```python
from build123d import *

# Parameters (mm, degrees)
SKETCH1_R           = 1.55
BOSS_EXTRUDE1_DEPTH = 4
SKETCH2_W           = 60
SKETCH2_H           = 8
BOSS_EXTRUDE2_DEPTH = 5


with BuildPart() as part:
    # Sketch1 → Boss-Extrude1 (new body)
    with BuildSketch(Plane.XY):
        Polygon((-30, 56), (-30, -56), (-10, -56), (-10, -36), (10, -36), (10, -56), (30, -56), (30, 56), align=None)
        with Locations((-20, -46)):
            Circle(SKETCH1_R, mode=Mode.SUBTRACT)
        with Locations((20, -46)):
            Circle(SKETCH1_R, mode=Mode.SUBTRACT)
        with Locations((-20, 46)):
            Circle(SKETCH1_R, mode=Mode.SUBTRACT)
        with Locations((20, 46)):
            Circle(SKETCH1_R, mode=Mode.SUBTRACT)
    extrude(amount=BOSS_EXTRUDE1_DEPTH)

    # Sketch2 → Boss-Extrude2 (add)
    with BuildSketch(Plane(origin=(0, 0, 0), x_dir=(-1, 0, 0), z_dir=(0, 0, -1))):
        with Locations((0, 32)):
            Rectangle(SKETCH2_W, SKETCH2_H)
        Polygon((30, -28), (-30, -28), (-30, -36), (-10, -36), (10, -36), (30, -36), align=None)
    extrude(amount=BOSS_EXTRUDE2_DEPTH)


solid = part.part
```
For this review, take the finished solid that the model builds, in its own axes (mm). A direction names the side the tool comes from. Round coordinates to 2 decimals unless told otherwise and drop trailing zeros. Order: outer loops, then holes, each group sorted by start corner. A loop starts at its lowest first (then second) coordinate and runs counter-clockwise, first axis right, second up. Notation, with made-up numbers: (86.5, 48) -> (110.5, 48) arc R22 ccw to (110.5, 65) -> close; hole circle Ø4 at (-35, 42.25). An arc over 180 degrees is marked (long way). Use a Markdown table: item, result.
Item 1: Machinability: for faces 4 (the flat face through (0, 36, -2)), 5 (the flat face through (0, -28, -2)), 6 (the flat face through (18, -46, 0)), 7 (the flat face through (-10, -46, 2)), which of the approach directions +Z, -Z, +X, -X, +Y, -Y give a long, thin tool a straight path to every point of the face, cutting with its end or side? Answer none if there is none.
Resolved:
| item | result |
|---|---|
| face 4 | -Z, +X, -X, +Y |
| face 5 | -Z, +X, -X |
| face 6 | -Z, +X, -X, -Y |
| face 7 | +Z, -Z, -Y |
Item 2: Take a section at B-B (x = -20). State the section outline as (y, z) points, plus the area to 3 significant figures.
Resolved:
| item | result |
|---|---|
| outline | (-56, 0) -> (-47.55, 0) -> (-47.55, 4) -> (-56, 4) -> close; (-44.45, 0) -> (-36, 0) -> (-36, -5) -> (-28, -5) -> (-28, 0) -> (28, 0) -> (28, -5) -> (36, -5) -> (36, 0) -> (44.45, 0) -> (44.45, 4) -> (-44.45, 4) -> close; (47.55, 0) -> (56, 0) -> (56, 4) -> (47.55, 4) -> close |
| area | 503 mm² |
Item 3: Take a section at A-A (z = -3). State the section outline as (x, y) points, plus the area to 3 significant figures.
Resolved:
| item | result |
|---|---|
| outline | (-30, -36) -> (30, -36) -> (30, -28) -> (-30, -28) -> close; (-30, 28) -> (30, 28) -> (30, 36) -> (-30, 36) -> close |
| area | 960 mm² |
Item 4: For pin 1 (5 mm diameter, centred on x = -20, y = -46, fed in from +Z); pin 2 (10 mm diameter, centred on x = 8.5, y = -4, fed in from -Z); pin 3 (2.5 mm diameter, centred on x = 4.5, z = -2, fed in from +Y); pin 4 (1.5 mm diameter, centred on x = 12, z = -3.5, fed in from -Y), all flat-tipped, find the tip position at first contact; note any pin that passes through.
Resolved:
| item | result |
|---|---|
| pin 1 | stops at z = 4 |
| pin 2 | stops at z = 0 |
| pin 3 | stops at y = 36 |
| pin 4 | stops at y = -36 |
Item 5: For line 1 along Y through (x, z) = (-20, 1.55); line 2 along Y through (x, z) = (-4.5, -1); line 3 along Z through (x, y) = (4.5, -22), list the stretches that pass through material, from the lowest coordinate up. Write a range as [from, to].
Resolved:
| item | result |
|---|---|
| line 1 | y = [-56, -47.55], [-44.45, 44.45], [47.55, 56] |
| line 2 | y = [-36, -28], [28, 36] |
| line 3 | z = [0, 4] |
Item 6: Take a section at D-D (z = 2.25). State the section outline as (x, y) points, plus the area to 3 significant figures.
Resolved:
| item | result |
|---|---|
| outline | (-30, -56) -> (-10, -56) -> (-10, -36) -> (10, -36) -> (10, -56) -> (30, -56) -> (30, 56) -> (-30, 56) -> close; hole circle Ø3.1 at (-20, -46); hole circle Ø3.1 at (-20, 46); hole circle Ø3.1 at (20, -46); hole circle Ø3.1 at (20, 46) |
| area | 6,290 mm² |
Item 7: Draft analysis for pull direction Y (two halves, no side actions). For faces 1 (the flat face through (0, 0, 0)), 2 (the flat face through (20, -56, 2)), 3 (the flat face through (0, 46, 0)), state which applies: +Y half, -Y half, draft (parallel to the pull), parting line (faces both ways), or undercut.
Resolved:
| item | result |
|---|---|
| face 1 | undercut |
| face 2 | -Y half |
| face 3 | draft |
Item 8: Take a section at C-C (y = -46). State the section outline as (x, z) points, plus the area to 3 significant figures.
Resolved:
| item | result |
|---|---|
| outline | (-30, 0) -> (-21.55, 0) -> (-21.55, 4) -> (-30, 4) -> close; (-18.45, 0) -> (-10, 0) -> (-10, 4) -> (-18.45, 4) -> close; (10, 0) -> (18.45, 0) -> (18.45, 4) -> (10, 4) -> close; (21.55, 0) -> (30, 0) -> (30, 4) -> (21.55, 4) -> close |
| area | 135 mm² |
